The figure shows three views and two pictorial views of one solid part (mm, origin at its lowest corner). Answer the questions. Give positions to 0.01 mm unless a question says otherwise; leave off trailing zeros. Loops run counter-clockwise (first coordinate to the right, second up) from the corner with the lowest first, then second, coordinate; pieces in that order, holes last. Notation, with made-up numbers: (-31, 61.25) -> (-12, 61.25) arc R14 ccw to (-12, 71.25) -> close; hole circle Ø1 at (43, 1). An arc over 180 degrees is marked (long way). Answer as CSV lines item,"result". Start each with the question number.
1. Find the intervals of material crossed by line 1 along X through (y, z) = (2.4, 127); line 2 along X through (y, z) = (5.4, 191), in increasing order.
2. Find section B-B, the plane z = 110.5. Give the vertices of the cut face in (x, y).
3. Find section A-A, the plane y = 1.7. Give the vertices of the cut face in (x, z), and give its area (3 significant figures).
4. Flat-ended cylindrical pins translate along their axes: pin 1 Ø3 at (y, z) = (3.5, 167) entering from +X; pin 2 Ø3 at (x, y) = (197, 2) entering from +Z; pin 3 Ø3 at (y, z) = (4, 117) entering from -X. Find the tip coordinate at first contact, or state that the pin passes through.
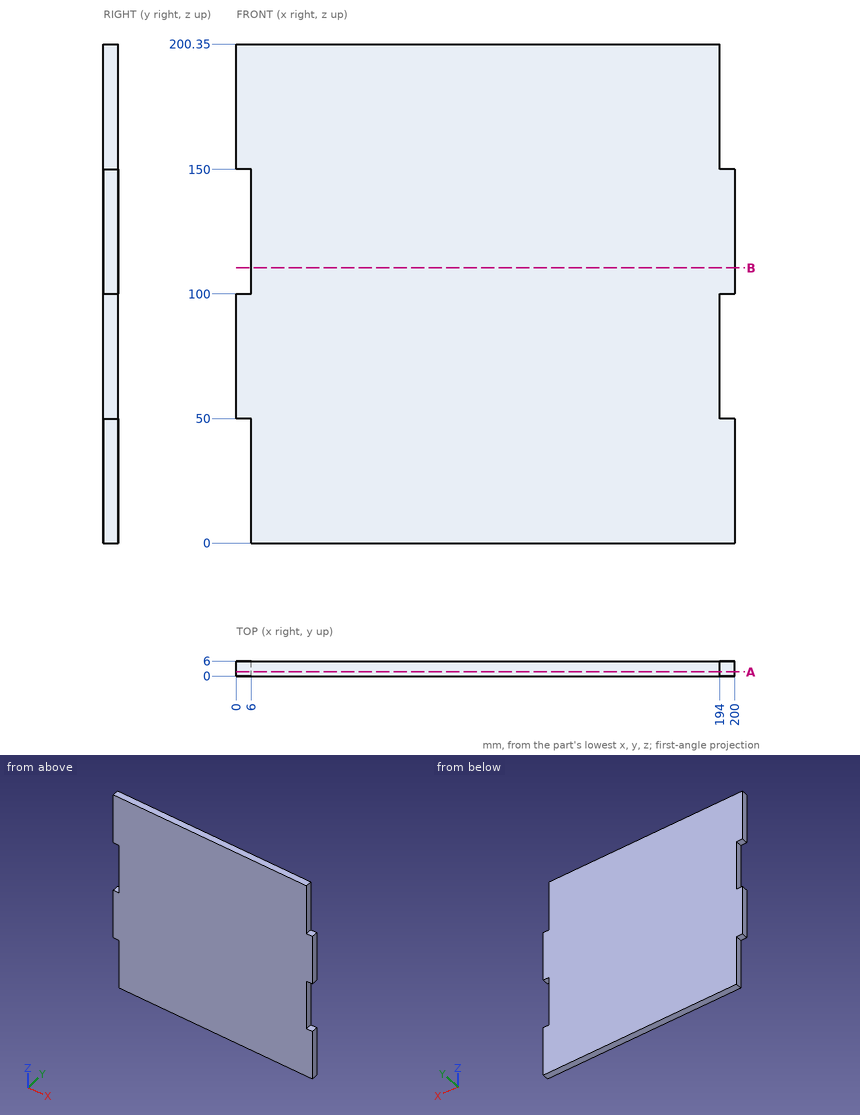
Resolved:
1,line 1,"x = 6 to 200"
1,line 2,"x = 0 to 194"
2,outline,"(6, 0) -> (200, 0) -> (200, 6) -> (6, 6) -> close"
3,outline,"(0, 50) -> (6, 50) -> (6, 0) -> (200, 0) -> (200, 50) -> (194, 50) -> (194, 100) -> (200, 100) -> (200, 150) -> (194, 150) -> (194, 200.35) -> (0, 200.35) -> (0, 150) -> (6, 150) -> (6, 100) -> (0, 100) -> close"
3,area,"38,900 mm^2"
4,pin 1,"stops at x = 194"
4,pin 2,"stops at z = 150"
4,pin 3,"stops at x = 6"
